Autodesk Inventor part; units mm, degrees
ref_plane "YZ Plane" through (0, 0, 0) normal (1, 0, 0) x (0, 1, 0)
ref_plane "XZ Plane" through (0, 0, 0) normal (0, 1, 0) x (-1, 0, 0)
ref_plane "XY Plane" through (0, 0, 0) normal (0, 0, 1) x (1, 0, 0)
sketch "Sketch1" plane through (0, 0, 0) normal (0, 1, 0) x (-1, 0, 0)
  line L0 (0, 0) -> (31.75, 0)
  line L1 (31.75, 0) -> (31.75, -31.75)
  line L2 (31.75, -31.75) -> (0, -31.75)
  line L3 (0, -31.75) -> (0, 0)
  line L4 (29.75, -29.75) -> (29.75, -2)
  line L5 (29.75, -2) -> (2, -2)
  line L6 (2, -2) -> (2, -29.75)
  line L7 (2, -29.75) -> (29.75, -29.75)
  dimension "d8" = 31.75
  dimension "d9" = 31.75
  dimension "d10" = 2
extrude "Extrusion1" add sketch "Sketch1" along normal blind 1310
sketch "Sketch3" plane through (-31.75, 0, 0) normal (0, 0, 1) x (1, 0, 0)
  line L0 (31.75, 0) -> (31.75, 368)
  line L1 (31.75, 0) -> (31.75, 1310)
  line L2 (0, 0) -> (31.75, 0)
  line L3 (31.75, 0) -> (31.75, 1310)
  line L4 (0, 1310) -> (31.75, 1310)
  line L5 (0, 0) -> (0, 1310)
  circle A0 centre (15.875, 375) radius 6
  circle A1 centre (15.875, 531) radius 6
  circle A2 centre (15.875, 687) radius 6
  circle A3 centre (15.875, 843) radius 6
  circle A4 centre (15.875, 999) radius 6
  circle A5 centre (15.875, 1155) radius 6
  dimension "d11" = 368
  dimension "d12" = 12
  dimension "d15" = 12
  dimension "d16" = 156
  dimension "d17" = 12
  dimension "d18" = 156
  dimension "d19" = 12
  dimension "d20" = 156
  dimension "d21" = 12
  dimension "d22" = 156
  dimension "d23" = 12
  dimension "d24" = 156
extrude "Extrusion2" cut sketch "Sketch3" against normal through all contours A0 | A1 | A2 | A3 | A4 | A5
sketch "Sketch4" plane through (0, 0, 0) normal (0, -1, 0) x (1, 0, 0)
  line L0 (0, -31.75) -> (-31.75, -31.75)
  line L1 (0, 0) -> (0, -31.75)
  line L2 (-31.75, 0) -> (0, 0)
  line L3 (-31.75, -31.75) -> (-31.75, 0)
  line L4 (-29.75, -29.75) -> (-2, -29.75)
  line L5 (-29.75, -2) -> (-29.75, -29.75)
  line L6 (-2, -2) -> (-29.75, -2)
  line L7 (-2, -29.75) -> (-2, -2)
  line L8 (0, 0) -> (30, 0)
  line L9 (30, 0) -> (30, -31.75)
  line L10 (30, -31.75) -> (0, -31.75)
  line L11 (0, -31.75) -> (0, 0)
  line L12 (-31.75, 0) -> (-61.75, 0)
  line L13 (-61.75, 0) -> (-61.75, -31.75)
  line L14 (-61.75, -31.75) -> (-31.75, -31.75)
  line L15 (-31.75, -31.75) -> (-31.75, 0)
  circle A0 centre (-46.75, -15.875) radius 6
  circle A1 centre (15, -15.875) radius 6
  dimension "d25" = 30
  dimension "d26" = 30
  dimension "d29" = 12
  dimension "d30" = 12
extrude "Extrusion3" add sketch "Sketch4" against normal blind 6 contours L1 L8 L9 L10 | L14 L13 L12 L3
sketch "Sketch5" plane through (0, 1310, 0) normal (0, 1, 0) x (1, 0, 0)
  line L0 (0, 31.75) -> (-31.75, 31.75)
  line L1 (30, 0) -> (-61.75, 0)
  line L2 (0, 31.75) -> (30, 31.75)
  line L3 (30, 31.75) -> (30, 0)
  line L4 (30, 0) -> (0, 0)
  line L5 (0, 0) -> (0, 31.75)
  line L6 (-31.75, 31.75) -> (-31.75, 0)
  line L7 (-61.75, 31.75) -> (-61.75, 0)
  line L8 (-31.75, 31.75) -> (-61.75, 31.75)
  line L9 (-61.75, 31.75) -> (-61.75, 0)
  line L10 (-61.75, 0) -> (-31.75, 0)
  line L11 (-31.75, 0) -> (-31.75, 31.75)
  circle A0 centre (-46.75, 15.875) radius 6
  circle A1 centre (-46.75, 15.875) radius 6
  circle A2 centre (15, 15.875) radius 6
  circle A3 centre (15, 15.875) radius 6
extrude "Extrusion4" add sketch "Sketch5" against normal blind 6 contours L2 L3 L1 L5 | L6 L1 L7 L8
sketch "Sketch6" plane through (-61.75, 0, 0) normal (0, 0, 1) x (1, 0, 0)
  circle A0 centre (45.875, 1274) radius 6
  line L0 (91.75, 1304) -> (61.75, 1304)
  circle A1 centre (45.875, 1212.25) radius 6
  point P0 (61.75, 0)
  dimension "d33" = 12
  dimension "d34" = 30
  dimension "d35" = 12
  dimension "d36" = 61.75
extrude "Extrusion5" cut sketch "Sketch6" against normal through all
sketch "Sketch7" plane through (-61.75, 0, 0) normal (0, 0, 1) x (1, 0, 0)
  circle A0 centre (45.875, 245) radius 6
  circle A1 centre (45.875, 375) radius 6
  point P0 (61.75, 0)
  dimension "d39" = 12
  dimension "d40" = 130
extrude "Extrusion6" cut sketch "Sketch7" against normal through all contours A0
properties part number "Perfil_Vertical_Acero"
CAD build for the part. Positions are in the model's coordinates, mm. A direction names the side the tool comes from. Give positions to 0.01 mm unless a question says otherwise; leave off trailing zeros. Loops run counter-clockwise (first coordinate to the right, second up) from the corner with the lowest first, then second, coordinate; pieces in that order, holes last. Notation, with made-up numbers: (-25.75, 31) - (19.25, 31) arc R36 ccw to (19.25, 70) - close; hole circle Ø6 at (9, 52). An arc over 180 degrees is marked (long way). Put each result on its own line as item: value.
Q1. Flat gauge pins, fed straight in: pin 1 (5 mm diameter, centred on y = 1011.5, z = -19, fed in from -X); pin 2 (12 mm diameter, centred on y = 1100, z = -16.5, fed in from +X). Where does each tip first touch, or does it go through?
Filled in:
pin 1: stops at x = -31.75
pin 2: stops at x = 0
Q2. Tool access for faces 1 (the face through (-15, 1310, -30)), 2 (the face through (-29.75, 646, -16)), 3 (the face through (-31.75, 646, -16)), 4 (the face through (8, 1304, -16)): list every direction of +Z, -Z, +X, -X, +Y, -Y with a clear straight run to the whole face (end or side of a thin tool).
Filled in:
face 1: +Z, -Z, +X, -X, +Y
face 2: +Y, -Y
face 3: +Z, -Z, -X
face 4: +Z, -Z, +X
Q3. Slice it at A-A (y = 332.5). Give the cut face in (x, z), plus the area to 3 significant figures.
Filled in:
outline: (-31.75, -31.75) - (0, -31.75) - (0, 0) - (-31.75, 0) - close; hole (-29.75, -29.75) - (-2, -29.75) - (-2, -2) - (-29.75, -2) - close
area: 238 mm²
Q4. Probe line 1 along Y through (x, z) = (4.5, -8); line 2 along X through (y, z) = (702, -11). List the from-to ranges inside material, lowest first.
Filled in:
line 1: y = 0 to 6, 1304 to 1310
line 2: x = -31.75 to -29.75, -2 to 0
Q5. Mould opens along Z. For faces 5 (the face through (-12, 652, 0)), 6 (the face through (-19, 652, -31.75)), 7 (the face through (-15, 0, -30)), 8 (the face through (-16, 646, -29.75)) say: pulls with the +Z half, pulls with the -Z half, needs draft (parallel to the pull), parting line crosses it, or undercut.
Filled in:
face 5: pulls with the +Z half
face 6: pulls with the -Z half
face 7: needs draft
face 8: undercut
